The figure shows three views and two pictorial views of one solid part (mm, origin at its lowest corner). Answer the questions. Coordinates: 2 decimals unless noted, no trailing zeros. Order: outer loops, then holes, each group sorted by start corner. A loop starts at its lowest first (then second) coordinate and runs counter-clockwise, first axis right, second up. Notation, with made-up numbers: (80.25, -17.75) -> (91.25, -17.75) arc R32 cw to (91.25, 13.25) -> close; hole circle Ø5 at (16, 72). An arc over 180 degrees is marked (long way). Write item = value, one per line.
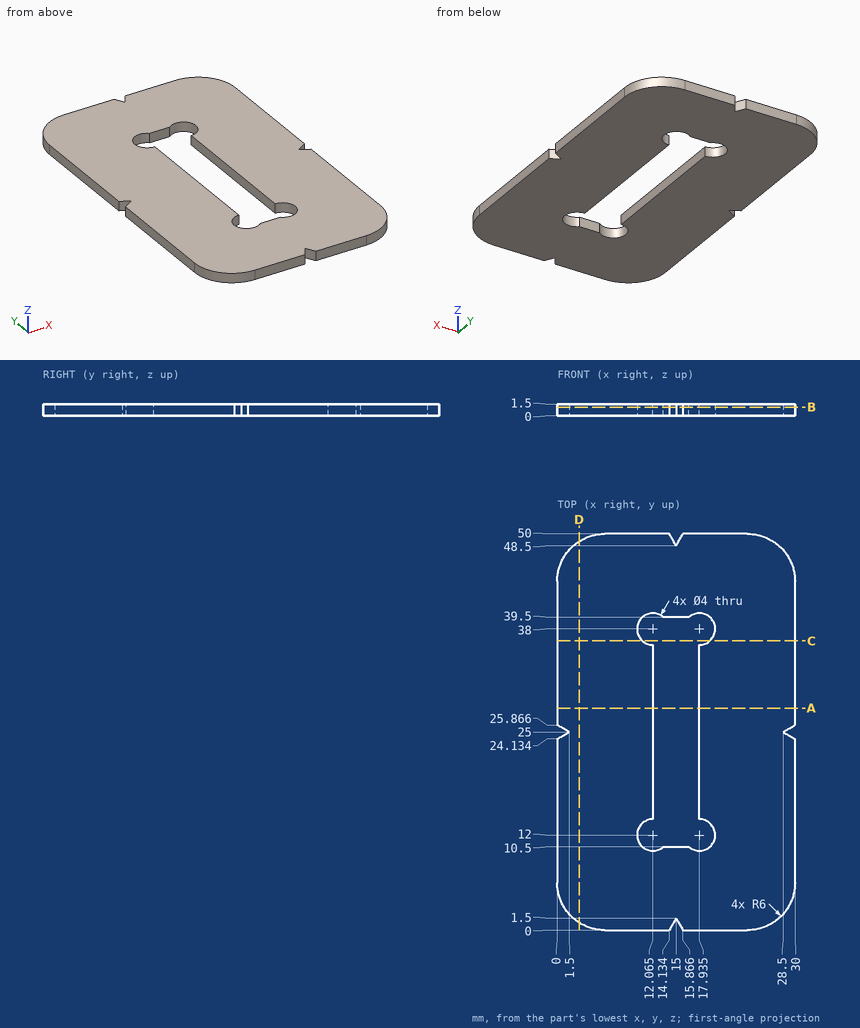
Q1. Section C-C, the plane y = 36.5 is taken. Give the vertices of the cut face in (x, z).
The answers:
outline = (0, 0) -> (10.74, 0) -> (10.74, 1.5) -> (0, 1.5) -> close; (19.26, 0) -> (30, 0) -> (30, 1.5) -> (19.26, 1.5) -> close
Q2. Section B-B, the plane z = 1.1 is taken. Give the vertices of the cut face in (x, y) (3 decimals).
The answers:
outline = (0, 6) arc R6 ccw to (6, 0) -> (14.134, 0) -> (15, 1.5) -> (15.866, 0) -> (24, 0) arc R6 ccw to (30, 6) -> (30, 24.134) -> (28.5, 25) -> (30, 25.866) -> (30, 44) arc R6 ccw to (24, 50) -> (15.866, 50) -> (15, 48.5) -> (14.134, 50) -> (6, 50) arc R6 ccw to (0, 44) -> (0, 25.866) -> (1.5, 25) -> (0, 24.134) -> close; hole (12.065, 14) arc R2 ccw (long way) to (13.388, 10.5) -> (16.612, 10.5) arc R2 ccw (long way) to (17.935, 14) -> (17.935, 36) arc R2 ccw (long way) to (16.612, 39.5) -> (13.388, 39.5) arc R2 ccw (long way) to (12.065, 36) -> close
Q3. Each of these flat-tipped pins is pushed along its axis until it touches: pin 1 Ø3 at (x, y) = (17.93, 38) entering from +Z; pin 2 Ø0.8 at (x, z) = (15, 1) entering from +Y. Where does it stop, or does it pass through?
The answers:
pin_1 = through
pin_2 = 49.19
Q4. Find the intervals of material crossed by line 1 along Y through (x, z) = (16, 0.35); line 2 along X through (y, z) = (19, 0.1) (3 decimals); line 3 along Y through (x, z) = (19, 0.45), in increasing order.
The answers:
line_1 = 0 to 10.5, 39.5 to 50
line_2 = 0 to 12.065, 17.935 to 30
line_3 = 0 to 10.31, 13.69 to 36.31, 39.69 to 50
Q5. Section D-D, the plane x = 2.75 is taken. Give the vertices of the cut face in (y, z), plus the area to 3 significant figures.
The answers:
outline = (0.96, 0) -> (49.04, 0) -> (49.04, 1.5) -> (0.96, 1.5) -> close
area = 72.1 mm2
Q6. Section A-A, the plane y = 28 is taken. Give the vertices of the cut face in (x, z) (3 decimals), plus the area to 3 significant figures.
The answers:
outline = (0, 0) -> (12.065, 0) -> (12.065, 1.5) -> (0, 1.5) -> close; (17.935, 0) -> (30, 0) -> (30, 1.5) -> (17.935, 1.5) -> close
area = 36.2 mm2
